from build123d import *

# Parameters (mm, degrees)
SKETCH1_R           = 11
BOSS_EXTRUDE1_DEPTH = 4.7625
SKETCH2_R           = 12
CUT_EXTRUDE1_DEPTH  = 6
SKETCH3_R           = 2.778125
CUT_EXTRUDE2_DEPTH  = 25.4


with BuildPart() as part:
    # Sketch1 → Boss-Extrude1 (new, symmetric)
    with BuildSketch(Plane(origin=(0, 0, 0), x_dir=(0, 0, -1), z_dir=(1, 0, 0))):
        Polygon((-38.1, -127), (-38.1, 15.781536726), (-15.781536726, 38.1), (15.781536726, 38.1), (38.1, 15.781536726), (38.1, -127), align=None)
        with Locations(Location((0, 0, 0), (0, 0, 180))):
            Circle(SKETCH1_R, mode=Mode.SUBTRACT)
    extrude(amount=BOSS_EXTRUDE1_DEPTH, both=True)

    # Sketch2 → Cut-Extrude1 (cut)
    with BuildSketch(Plane(origin=(4.7625, 0, 0), x_dir=(0, 0, -1), z_dir=(1, 0, 0))):
        Circle(SKETCH2_R)
    extrude(amount=-CUT_EXTRUDE1_DEPTH, mode=Mode.SUBTRACT)

    # Sketch3 → Cut-Extrude2 (cut)
    with BuildSketch(Plane.XZ.offset(127)):
        with Locations(Location((0, 30.1625, 0), (0, 0, 270))):
            Circle(SKETCH3_R)
        with Locations(Location((0, -30.1625, 0), (0, 0, 270))):
            Circle(SKETCH3_R)
    extrude(amount=-CUT_EXTRUDE2_DEPTH, mode=Mode.SUBTRACT)


solid = part.part
Design review of the part built by this model. Coordinates are the model's own, in mm. A direction names the side the tool comes from. Round coordinates to 2 decimals unless told otherwise and drop trailing zeros. Write each loop counter-clockwise with the first axis right and the second up, starting at its lowest first coordinate (ties: lowest second). Pieces come first, ordered by that corner, then holes. Notation, with made-up numbers: (43.5, 42.5) - (63.5, 42.5) arc R13 cw to (63.5, 48.5) - close; hole circle Ø9 at (14, -20). An arc over 180 degrees is marked (long way). Return JSON: item names as keys, results as strings. Group by question number.
Item 1: We need section C-C on y = -109.5. Write out the cut boundary in (x, z).
Item 2: The part is to be moulded in two halves that separate along Z. For faces 4 (the face through (-1.237, -10, -5)), 5 (the face through (0, -57, 38.1)), 6 (the face through (4.762, -43, -1)), say which applies: pulls with the +Z half, pulls with the -Z half, needs draft (parallel to the pull), parting line crosses it, or undercut.
Item 3: Insertion check: P1, Ø19, axis at y = 0, z = 0, coming from the -X side; P2, Ø4, axis at x = -2.5, z = -20.5, coming from the +Y side; P3, Ø5, axis at x = 0, z = 30.16, coming from the +Y side; P4, Ø12, axis at y = -0.5, z = 5.5, coming from the +X side. Each pin has a flat end and moves straight along its axis. Give the tip position at first contact, or say it passes through.
Item 4: Machinability: for faces 1 (the face through (1.8, 0.53, 11.99)), 2 (the face through (0.122, -114.478, -27.387)), 3 (the face through (0, 38.1, 0)), which of the approach directions +Z, -Z, +X, -X, +Y, -Y give a long, thin tool a straight path to every point of the face, cutting with its end or side? Answer none if there is none.
Item 5: We need section A-A on z = 0. Write out the cut boundary in (x, y).
Item 6: We need section B-B on y = 0. Write out the cut boundary in (x, z), and give its area (3 significant figures).
Item 7: For probe 1 along Y at (x, z) = (0.85, 0); probe 2 along Y at (x, z) = (-2.6, 0); probe 3 along Z at (x, y) = (2.25, -2), list the stretches that pass through material, from the lowest coordinate up. Write a range as [from, to].
Item 8: We need section D-D on y = 18.5. Write out the cut boundary in (x, z).
Model answer:
{
 "1": {"outline": "(-4.76, -38.1) - (4.76, -38.1) - (4.76, 38.1) - (-4.76, 38.1) - close; hole circle Ø5.56 at (0, -30.16); hole circle Ø5.56 at (0, 30.16)"},
 "2": {"face 4": "undercut", "face 5": "pulls with the +Z half", "face 6": "needs draft"},
 "3": {"P1": "passes through", "P2": "stops at y = 35.38", "P3": "stops at y = 26.22", "P4": "stops at x = -1.24"},
 "4": {"face 1": "+X", "face 2": "-Y", "face 3": "+Z, -Z, +X, -X, +Y"},
 "5": {"outline": "(-4.76, -127) - (4.76, -127) - (4.76, -12) - (-1.24, -12) - (-1.24, -11) - (-4.76, -11) - close; (-4.76, 11) - (-1.24, 11) - (-1.24, 12) - (4.76, 12) - (4.76, 38.1) - (-4.76, 38.1) - close"},
 "6": {"outline": "(-4.76, -38.1) - (4.76, -38.1) - (4.76, -12) - (-1.24, -12) - (-1.24, -11) - (-4.76, -11) - close; (-4.76, 11) - (-1.24, 11) - (-1.24, 12) - (4.76, 12) - (4.76, 38.1) - (-4.76, 38.1) - close", "area": "504 mm²"},
 "7": {"probe 1": "y = [-127, -12], [12, 38.1]", "probe 2": "y = [-127, -11], [11, 38.1]", "probe 3": "z = [-38.1, -11.83], [11.83, 38.1]"},
 "8": {"outline": "(-4.76, -35.38) - (4.76, -35.38) - (4.76, 35.38) - (-4.76, 35.38) - close"}
}
